Can you work these out from the drawing? Everything is in mm from the part's minimum corner. Give positions to 0.01 mm unless a question says otherwise; leave off trailing zeros. Loops run counter-clockwise (first coordinate to the right, second up) from the corner with the lowest first, then second, coordinate; pieces in that order, holes last.
Q1. If we section it at D-D (x = 53): Please give me the cut outline in (y, z), plus the area to 3 significant figures.
Q2. I need wall thicknesses on line 1 (Y direction, x = 66.5, z = 0.75); line 2 (Y direction, x = 53, z = 1.1); line 3 (X direction, y = 97.5, z = 1.05). Which ranges of each line are inside material? Lowest first, please.
Q3. If we section it at C-C (z = 2.4): Give the number of separate pieces and of enclosed holes in the cut face, plus the area to 3 significant figures.
Q4. If we section it at B-B (y = 97.5): Please give me the cut outline in (x, z).
Q5. Will this pin go through, and if not, where does the flat tip stop? P1, Ø5, axis at x = 21, y = 56.5, coming from the +Z side.
Q6. If we section it at A-A (x = 66.5): Please give me the cut outline in (y, z), plus the area to 3 significant figures.
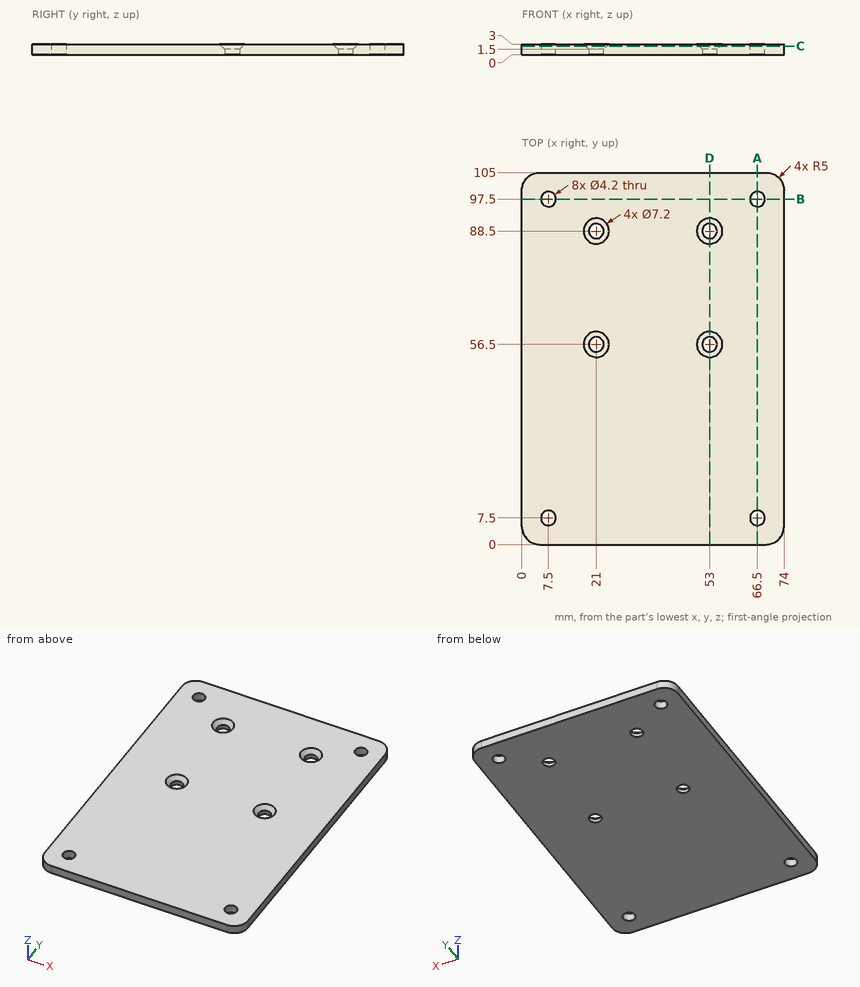
Check sheet entries:
1. outline: (0, 0) - (54.4, 0) - (54.4, 1.5) - (52.9, 3) - (0, 3) - close; (58.6, 0) - (86.4, 0) - (86.4, 1.5) - (84.9, 3) - (60.1, 3) - (58.6, 1.5) - close; (90.6, 0) - (105, 0) - (105, 3) - (92.1, 3) - (90.6, 1.5) - close
1. area: 285 mm2
2. line 1: y = 0 to 5.4, 9.6 to 95.4, 99.6 to 105
2. line 2: y = 0 to 54.4, 58.6 to 86.4, 90.6 to 105
2. line 3: x = 0 to 5.4, 9.6 to 64.4, 68.6 to 74
3. separate pieces: 1
3. enclosed holes: 8
3. area: 7,580 mm2
4. outline: (0, 0) - (5.4, 0) - (5.4, 3) - (0, 3) - close; (9.6, 0) - (64.4, 0) - (64.4, 3) - (9.6, 3) - close; (68.6, 0) - (74, 0) - (74, 3) - (68.6, 3) - close
5. P1: stops at z = 1.9
6. outline: (0, 0) - (5.4, 0) - (5.4, 3) - (0, 3) - close; (9.6, 0) - (95.4, 0) - (95.4, 3) - (9.6, 3) - close; (99.6, 0) - (105, 0) - (105, 3) - (99.6, 3) - close
6. area: 290 mm2
